from build123d import *

# Parameters (mm, degrees)
F1_DEPTH = 2.5


with BuildPart() as f1:
    # F0 (on Front) → F1 (new body)
    with BuildSketch(Plane.XZ):
        Polygon((42.389926, 8.394053), (-9.838827, 97.432958), (-62.206484, 8.394053), align=None)
        Polygon((16.607858, 45.820797), (36.624869, 11.696054), (-6.56895, 11.696054), (-7.898982, 11.696054), (-11.791403, 11.696054), (-12.757268, 11.696054), (-56.433667, 11.696054), (-35.484269, 47.315586), (-29.714779, 57.12525), (-11.791403, 87.599742), (-9.842608, 90.91321), (-7.898982, 87.599742), (9.345976, 58.20076), align=None, mode=Mode.SUBTRACT)
        with BuildLine():
            Line((-12.757268, 11.696054), (-11.791403, 11.696054))
            Line((-11.791403, 11.696054), (-11.791403, 14.763876))
            ThreePointArc((-11.791403, 14.763876), (-33.72406, 38.730513), (-11.791403, 62.697151))
            Line((-11.791403, 62.697151), (-11.791403, 65.858104))
            ThreePointArc((-11.791403, 65.858104), (-21.581724, 63.19237), (-29.714779, 57.12525))
            Line((-29.714779, 57.12525), (-35.484269, 47.315586))
            ThreePointArc((-35.484269, 47.315586), (-32.602413, 24.094116), (-12.757268, 11.696054))
        make_face()
        Polygon((-11.791403, 11.696054), (-7.898982, 11.696054), (-7.898982, 14.734322), (-7.898982, 62.726705), (-7.898982, 65.884218), (-7.898982, 87.599742), (-9.842608, 90.91321), (-11.791403, 87.599742), (-11.791403, 65.858104), (-11.791403, 62.697151), (-11.791403, 14.763876), align=None)
        with BuildLine():
            ThreePointArc((-6.56895, 11.696054), (12.846937, 23.442164), (16.607858, 45.820797))
            Line((16.607858, 45.820797), (9.345976, 58.20076))
            ThreePointArc((9.345976, 58.20076), (1.411206, 63.586003), (-7.898982, 65.884218))
            Line((-7.898982, 65.884218), (-7.898982, 62.726705))
            ThreePointArc((-7.898982, 62.726705), (14.397842, 38.730513), (-7.898982, 14.734322))
            Line((-7.898982, 14.734322), (-7.898982, 11.696054))
            Line((-7.898982, 11.696054), (-6.56895, 11.696054))
        make_face()
    extrude(amount=F1_DEPTH)


solid = f1.part
The model under review builds one solid part; all positions refer to its coordinate system, in mm. A direction names the side the tool comes from. Round coordinates to 2 decimals unless told otherwise and drop trailing zeros. Loops run counter-clockwise (first coordinate to the right, second up) from the corner with the lowest first, then second, coordinate; pieces in that order, holes last. Notation, with made-up numbers: M 14,56 L 31,56 A29 cw 31,84 Z; hole C -38.5,15.25 d5. An arc over 180 degrees is marked long. Answer as CSV lines item,"result".
1. We need section B-B (z = 19). Give the boundary of the cut face in (x, y).
Outcome:
outline,"M -55.97,-2.5 L -52.14,-2.5 L -52.14,0 L -55.97,0 Z; M -28.4,-2.5 L -23.43,-2.5 L -23.43,0 L -28.4,0 Z; M -11.79,-2.5 L -7.9,-2.5 L -7.9,0 L -11.79,0 Z; M 4.11,-2.5 L 9.08,-2.5 L 9.08,0 L 4.11,0 Z; M 32.34,-2.5 L 36.17,-2.5 L 36.17,0 L 32.34,0 Z"
2. To check wall thickness, follow L1, parallel to X at y = -1.45, z = 67.5; L2, parallel to X at y = -0.35, z = 54; L3, parallel to Z at x = -3, y = -2. State the ranges of each line that lie inside material, in increasing order. Write a range as [from, to].
Outcome:
L1,"x = [-27.44, -23.61], [-11.79, -7.9], [3.89, 7.72]"
L2,"x = [-35.38, -28.26], [-11.79, -7.9], [8.93, 15.64]"
L3,"z = [8.39, 11.7], [12.35, 15.61], [61.85, 65.11], [79.25, 85.77]"
3. We need section A-A (x = 22). Give the boundary of the cut face in (y, z).
Outcome:
outline,"M -2.5,8.39 L 0,8.39 L 0,11.7 L -2.5,11.7 Z; M -2.5,36.63 L 0,36.63 L 0,43.15 L -2.5,43.15 Z"
4. We need section C-C (y = -1.45). Give the boundary of the cut face in (x, z).
Outcome:
outline,"M -62.21,8.39 L 42.39,8.39 L -9.84,97.43 Z; hole M -56.43,11.7 L -12.76,11.7 A27.21 cw -35.48,47.32 Z; hole M -29.71,57.13 A27.21 cw -11.79,65.86 L -11.79,87.6 Z; hole M -11.79,14.76 L -11.79,62.7 A24.06 ccw Z; hole M -7.9,14.73 A24.06 ccw -7.9,62.73 Z; hole M -7.9,65.88 A27.21 cw 9.35,58.2 L -7.9,87.6 Z; hole M -6.57,11.7 L 36.62,11.7 L 16.61,45.82 A27.21 cw Z"
5. For faces 1 (the face through (-11.791, -1, 39)), 2 (the face through (-10, -2.5, 40)), list the 3-axis set-ups (+Z, -Z, +X, -X, +Y, -Y) from which the entire face can be reached by the end or side of a thin tool; tool diameter is ignored.
Outcome:
face 1,"+Y, -Y"
face 2,"+Z, -Z, +X, -X, -Y"
6. We need section D-D (z = 68). Give the boundary of the cut face in (x, y).
Outcome:
outline,"M -27.15,-2.5 L -23.32,-2.5 L -23.32,0 L -27.15,0 Z; M -11.79,-2.5 L -7.9,-2.5 L -7.9,0 L -11.79,0 Z; M 3.6,-2.5 L 7.43,-2.5 L 7.43,0 L 3.6,0 Z"
7. Draft analysis for pull direction Z (two halves, no side actions). For faces 3 (the face through (-46.106, -1.232, 29.256)), 4 (the face through (-11, -1, 8.394)), 5 (the face through (-34, -1, 11.696)), 6 (the face through (-10, 0, 40)), state which applies: pulls with the +Z half, pulls with the -Z half, needs draft (parallel to the pull), parting line crosses it, or undercut.
Outcome:
face 3,"undercut"
face 4,"pulls with the -Z half"
face 5,"undercut"
face 6,"needs draft"
8. Insertion check: pin 1 Ø1.5 at (y, z) = (-2, 23) entering from +X; pin 2 Ø1.2 at (y, z) = (-1, 75.5) entering from +X; pin 3 Ø1.2 at (x, y) = (9.5, -1.5) entering from +Z. Each pin has a flat end and moves straight along its axis. Give the tip position at first contact, or say it passes through.
Outcome:
pin 1,"stops at x = 34.26"
pin 2,"stops at x = 3.38"
pin 3,"stops at z = 65.49"
